CAD build for the part. Positions are in the model's coordinates, mm. A direction names the side the tool comes from. Give positions to 0.01 mm unless a question says otherwise; leave off trailing zeros. Loops run counter-clockwise (first coordinate to the right, second up) from the corner with the lowest first, then second, coordinate; pieces in that order, holes last.
```python
from build123d import *

# Parameters (mm, degrees)
F0_W         = 76.2
F0_H         = 127
F1_DEPTH     = 139.7
F2_R         = 11.43
F3_DEPTH     = 91.44
F4_R         = 10.16
F5_DEPTH     = 133.35
F6_DEPTH     = 12.7
F8_DEPTH     = 5.08
F7_W         = 60.1533111874
F7_H         = 25.4809018224
F7_W_2       = 0.8066888126
F9_DEPTH     = 63.5
F10_DEPTH    = 91.44
F11_R        = 11.43
F12_DEPTH    = 91.44
F13_W        = 60.96
F13_H        = 20.32
F14_DEPTH    = 88.9
F15_DEPTH    = 5.08
F16_DEPTH    = 5.08
F17_W        = 50.8
F17_H        = 12.7
F18_DEPTH    = 86.36
F19_W        = 50.8
F19_H        = 48.0175957203
F20_DEPTH    = 88.9
F21_W        = 6.7573417909
F21_H        = 48.0175957203
F22_DEPTH    = 55.88
F23_W        = 60.96
F23_H        = 38.1
F24_DEPTH    = 38.1
F25_W        = 34.0146065784
F25_H        = 50.826728344
F26_DEPTH    = 50.8
F27_T1_DEPTH = 38.1
F28_DEPTH    = 0.508
F29_DEPTH    = 0.508
F30_DEPTH    = 0.508
F31_DEPTH    = 0.381
F32_DEPTH    = 25.4


# Not quite as in the source:
# - a fillet or chamfer that OpenCascade refuses, or shapes differently, is made with other operations: its cross-section is extruded or revolved along the edge and cut away or added


with BuildPart() as f1:
    # F0 (on Top) → F1 (new body)
    with BuildSketch(Plane.XY):
        with Locations((38.1, 63.5)):
            Rectangle(F0_W, F0_H)
    extrude(amount=F1_DEPTH)

    # F2 (on face) → F3 (cut)
    with BuildSketch(Plane.XY.offset(139.7)):
        with Locations((18.5702368617, 17.6018252969)):
            Circle(F2_R)
    extrude(amount=-F3_DEPTH, mode=Mode.SUBTRACT)

    # F4 (on face) → F5 (cut)
    with BuildSketch(Plane.XY.offset(139.7)):
        with Locations((20.5664373934, 108.7463870645)):
            Circle(F4_R)
    extrude(amount=-F5_DEPTH, mode=Mode.SUBTRACT)

    # F6 (cut): a face of the model
    f6_faces = [f1.faces().sort_by_distance(p)[0] for p in [
        (76.2, 63.5, 69.85),
    ]]
    extrude(f6_faces, amount=-F6_DEPTH, mode=Mode.SUBTRACT)

    # F8 (add): a face of the model
    f8_faces = [f1.faces().sort_by_distance(p)[0] for p in [
        (63.5, 63.5, 69.85),
    ]]
    extrude(f8_faces, amount=F8_DEPTH)

    # F7 (on face) → F9 (cut)
    with BuildSketch(Plane.XZ):
        with Locations((33.4233444063, 16.9386500493)):
            Rectangle(F7_W, F7_H)
        with Locations((63.9033444063, 16.9386500493)):
            Rectangle(F7_W_2, F7_H)
    extrude(amount=-F9_DEPTH, mode=Mode.SUBTRACT)

    # F10 (add): a face of the model
    f10_faces = [f1.faces().sort_by_distance(p)[0] for p in [
        (18.5702368617, 17.6018252969, 48.26),
    ]]
    extrude(f10_faces, amount=F10_DEPTH)

    # F11 (on face) → F12 (cut)
    with BuildSketch(Plane.XY.offset(139.7)):
        with Locations((49.913611263, 109.6450760961)):
            Circle(F11_R)
    extrude(amount=-F12_DEPTH, mode=Mode.SUBTRACT)

    # F13 (on face) → F14 (cut)
    with BuildSketch(Plane.XZ):
        with Locations((33.8266888126, 53.3226364589)):
            Rectangle(F13_W, F13_H)
    extrude(amount=-F14_DEPTH, mode=Mode.SUBTRACT)

    # F15 (add): a face of the model
    f15_faces = [f1.faces().sort_by_distance(p)[0] for p in [
        (3.3466888126, 44.45, 53.3226364589),
    ]]
    extrude(f15_faces, amount=F15_DEPTH)

    # F16 (add): a face of the model
    f16_faces = [f1.faces().sort_by_distance(p)[0] for p in [
        (64.3066888126, 44.45, 53.3226364589),
    ]]
    extrude(f16_faces, amount=F16_DEPTH)

    # F17 (on face) → F18 (cut)
    with BuildSketch(Plane.XZ):
        with Locations((33.8266888126, 78.1391007662)):
            Rectangle(F17_W, F17_H)
    extrude(amount=-F18_DEPTH, mode=Mode.SUBTRACT)

    # F19 (on face) → F20 (cut)
    with BuildSketch(Plane.XZ):
        with Locations((33.8266888126, 115.6912021399)):
            Rectangle(F19_W, F19_H)
    extrude(amount=-F20_DEPTH, mode=Mode.SUBTRACT)

    # F21 (on face) → F22 (join)
    with BuildSketch(Plane.YZ.offset(8.4266888126)):
        with Locations((3.3786708955, 115.6912021399)):
            Rectangle(F21_W, F21_H)
    extrude(amount=F22_DEPTH)

    # F23 (on face) → F24 (join)
    with BuildSketch(Plane.YZ.offset(68.58)):
        with Locations((96.52, 120.65)):
            Rectangle(F23_W, F23_H)
    extrude(amount=F24_DEPTH)

    # F25 (on face) → F26 (cut)
    with BuildSketch(Plane(origin=(0, 0, 101.6), x_dir=(1, 0, 0), z_dir=(0, 0, -1))):
        with Locations((85.5873032892, -96.4670181274)):
            Rectangle(F25_W, F25_H)
    extrude(amount=-F26_DEPTH, mode=Mode.SUBTRACT)

    # F27: fillet of radius 25.4 on 4 edges, made by hand

    # F27_s2 → F27_t1 (join)
    with BuildSketch(Plane.XY.offset(101.6)):
        with BuildLine():
            ThreePointArc((77.1946065784, 71.0536539555), (95.1551188205, 78.4931417133), (102.5946065784, 96.4536539555))
            Line((102.5946065784, 96.4536539555), (102.5946065784, 71.0536539555))
            Line((102.5946065784, 71.0536539555), (77.1946065784, 71.0536539555))
        make_face()
        with BuildLine():
            ThreePointArc((102.5946065784, 96.4803822994), (95.1551188205, 114.4408945416), (77.1946065784, 121.8803822994))
            Line((77.1946065784, 121.8803822994), (102.5946065784, 121.8803822994))
            Line((102.5946065784, 121.8803822994), (102.5946065784, 96.4803822994))
        make_face()
        with BuildLine():
            ThreePointArc((68.58, 96.4536539555), (76.0194877579, 78.4931417133), (93.98, 71.0536539555))
            Line((93.98, 71.0536539555), (68.58, 71.0536539555))
            Line((68.58, 71.0536539555), (68.58, 96.4536539555))
        make_face()
        with BuildLine():
            ThreePointArc((68.58, 96.4803822994), (76.0194877579, 114.4408945416), (93.98, 121.8803822994))
            Line((93.98, 121.8803822994), (68.58, 121.8803822994))
            Line((68.58, 121.8803822994), (68.58, 96.4803822994))
        make_face()
    extrude(amount=F27_T1_DEPTH)

    # F28 (cut): a face of the model
    f28_faces = [f1.faces().sort_by_distance(p)[0] for p in [
        (33.8266888126, 63.5, 16.9386500493),
    ]]
    extrude(f28_faces, amount=-F28_DEPTH, mode=Mode.SUBTRACT)

    # F29 (cut): a face of the model
    f29_faces = [f1.faces().sort_by_distance(p)[0] for p in [
        (3.3466888126, 32.004, 16.9386500493),
    ]]
    extrude(f29_faces, amount=-F29_DEPTH, mode=Mode.SUBTRACT)

    # F30 (cut): a face of the model
    f30_faces = [f1.faces().sort_by_distance(p)[0] for p in [
        (64.3066888126, 32.004, 16.9386500493),
    ]]
    extrude(f30_faces, amount=-F30_DEPTH, mode=Mode.SUBTRACT)

    # F31 (cut): a face of the model
    f31_faces = [f1.faces().sort_by_distance(p)[0] for p in [
        (33.8266888126, 43.18, 84.4891007662),
    ]]
    extrude(f31_faces, amount=-F31_DEPTH, mode=Mode.SUBTRACT)

    # F32 (cut): a face of the model
    f32_faces = [f1.faces().sort_by_distance(p)[0] for p in [
        (33.8266888126, 6.7573417909, 115.6912021399),
    ]]
    extrude(f32_faces, amount=-F32_DEPTH, mode=Mode.SUBTRACT)


solid = f1.part
```
1. Saw through at B-B, the plane x = 72. List the corners of the cut face in (y, z), and give its area (3 significant figures).
Responses:
outline: (66.04, 101.6) - (83.72, 101.6) - (83.72, 139.7) - (66.04, 139.7) - close; (109.21, 101.6) - (127, 101.6) - (127, 139.7) - (109.21, 139.7) - close
area: 1,350 mm2
2. Saw through at A-A, the plane y = 35.5. List the corners of the cut face in (x, z).
Responses:
outline: (0, 0) - (68.58, 0) - (68.58, 139.7) - (59.23, 139.7) - (59.23, 91.68) - (8.43, 91.68) - (8.43, 139.7) - (0, 139.7) - close; hole (2.84, 4.2) - (64.81, 4.2) - (64.81, 29.68) - (2.84, 29.68) - close; hole (8.43, 43.16) - (59.23, 43.16) - (59.23, 63.48) - (8.43, 63.48) - close; hole (8.43, 71.79) - (59.23, 71.79) - (59.23, 84.87) - (8.43, 84.87) - close
3. Saw through at C-C, the plane y = 102. List the corners of the cut face in (x, z).
Responses:
outline: (0, 0) - (68.58, 0) - (68.58, 101.6) - (69.19, 101.6) - (69.19, 139.7) - (58.41, 139.7) - (58.41, 48.26) - (41.42, 48.26) - (41.42, 139.7) - (28.16, 139.7) - (28.16, 6.35) - (12.97, 6.35) - (12.97, 139.7) - (0, 139.7) - close; (101.99, 101.6) - (106.68, 101.6) - (106.68, 139.7) - (101.99, 139.7) - close
4. Pull direction Y, two halves, no side cores. Call faces 5 (the face through (73.137, 81.936, 120.383)), 6 (the face through (33, 88.9, 53)), 7 (the face through (59.227, 44, 53)), 8 (the face through (47.436, 98.487, 94.62)): released by +Y, released by -Y, zero draft, split by the parting line, or undercut.
Responses:
face 5: undercut
face 6: released by -Y
face 7: zero draft
face 8: undercut
5. Probe line 1 along Z through (x, y) = (29, 45); line 2 along X through (y, z) = (51, 122.5); line 3 along X through (y, z) = (102.5, 67). List the from-to ranges inside material, lowest first.
Responses:
line 1: z = 0 to 4.2, 29.68 to 43.16, 63.48 to 71.79, 84.87 to 91.68
line 2: x = 0 to 8.43, 59.23 to 68.58
line 3: x = 0 to 12.55, 28.58 to 40.99, 58.84 to 68.58
6. Saw through at D-D, the plane z = 46.5. List the corners of the cut face in (x, y), and give its area (3 significant figures).
Responses:
outline: (0, 0) - (8.43, 0) - (8.43, 88.9) - (59.23, 88.9) - (59.23, 0) - (68.58, 0) - (68.58, 127) - (0, 127) - close; hole circle Ø20.32 at (20.57, 108.75)
area: 3,870 mm2
7. Drop flat-ended pins along their axis: pin 1 (10 mm diameter, centred on x = 21.5, y = 111, fed in from +Z); pin 2 (11.5 mm diameter, centred on x = 90, y = 84, fed in from -Z); pin 3 (6 mm diameter, centred on y = 50, z = 95.5, fed in from +X); pin 4 (8 mm diameter, centred on x = 20, y = 51, fed in from +Z). Give the stop position or say it passes through.
Responses:
pin 1: stops at z = 6.35
pin 2: passes through
pin 3: stops at x = 68.58
pin 4: stops at z = 91.68
8. Tool access for faces 1 (the face through (50, 110, 48.26)), 2 (the face through (105, 97, 101.6)), 3 (the face through (34, 32, 4.198)), 4 (the face through (8.427, 45, 115)): list every direction of +Z, -Z, +X, -X, +Y, -Y with a clear straight run to the whole face (end or side of a thin tool).
Responses:
face 1: +Z
face 2: -Z, +X, +Y, -Y
face 3: -Y
face 4: +Z, -Y
